```python
from build123d import *

# Parameters (mm, degrees)
F1_DEPTH  = 9.398
F1_FACE_W = 97.914338
F1_FACE_H = 9.398
F2_DEPTH  = 25.4


with BuildPart() as f1:
    # F0 (on Top) → F1 (new body)
    with BuildSketch(Plane.XY):
        Polygon((40.420551, 41.290432), (-57.493787, 42.872965), (-57.493787, -29.132366), (40.420551, -29.132366), (40.420551, 27.838886), align=None)
        Polygon((-53.017702, -20.82406), (-53.017702, 36.542833), (34.834471, 34.169026), (34.834471, -22.243964), align=None, mode=Mode.SUBTRACT)
    extrude(amount=-F1_DEPTH)

    # F1_face (on face) → F2 (join)
    with BuildSketch(Plane(origin=(-8.536618, -29.132366, -4.699), x_dir=(1, 0, 0), z_dir=(0, -1, 0))):
        Rectangle(F1_FACE_W, F1_FACE_H)
    extrude(amount=F2_DEPTH)


solid = f1.part
```
Design review of the part built by this model. Coordinates are the model's own, in mm. A direction names the side the tool comes from. Round coordinates to 2 decimals unless told otherwise and drop trailing zeros. Write each loop counter-clockwise with the first axis right and the second up, starting at its lowest first coordinate (ties: lowest second). Pieces come first, ordered by that corner, then holes. Notation, with made-up numbers: (86, 64.25) -> (106, 64.25) arc R27 ccw to (106, 81.25) -> close; hole circle Ø11 at (-5.75, 29.5). An arc over 180 degrees is marked (long way). Write item = value, one per line. Start each with the question number.
1) Mouldability with a two-part tool opening along Y and no side actions: class faces 3 (the face through (-57.494, -5, -5)), 4 (the face through (-9, -54.532, -5)), 5 (the face through (-53.018, 7, -5)) as +Y half, -Y half, draft (parallel to the pull), parting line (faces both ways), or undercut.
2) Take a section at A-A, the plane z = -2. State the section outline as (x, y) points.
3) Clearance check with flat-ended pins moving along their axes: pin 1 (2 mm diameter, centred on x = 28, z = -3.5, fed in from +Y); pin 2 (5 mm diameter, centred on x = -44, y = -18, fed in from -Z). State where each tip first meets the part, or that it passes through.
4) Tool access review of faces 1 (the face through (34.834, 6, -5)), 2 (the face through (40.421, -6, -5)): name each direction out of +Z, -Z, +X, -X, +Y, -Y from which nothing blocks a thin tool from reaching the whole face with its end or side.
5) Wall thickness on probe 1 along X at (y, z) = (12.5, -8.5); probe 2 along Y at (x, z) = (32.5, -1.5); probe 3 along Y at (x, z) = (29, -3): over which ranges is each line inside the solid? List them lowest first. Write a range as from..to.
6) Take a section at C-C, the plane x = 10. State the section outline as (y, z) points, plus the area to 3 significant figures.
7) Take a section at B-B, the plane y = 10. State the section outline as (x, z) points, plus the area to 3 significant figures.
Results list:
q1.face_3 = draft
q1.face_4 = -Y half
q1.face_5 = undercut
q2.outline = (-57.49, -54.53) -> (40.42, -54.53) -> (40.42, 41.29) -> (-57.49, 42.87) -> close; hole (-53.02, -20.82) -> (34.83, -22.24) -> (34.83, 34.17) -> (-53.02, 36.54) -> close
q3.pin_1 = 41.51
q3.pin_2 = through
q4.face_1 = +Z, -Z
q4.face_2 = +Z, -Z, +X, +Y, -Y
q5.probe_1 = -57.49..-53.02, 34.83..40.42
q5.probe_2 = -54.53..-22.21, 34.23..41.42
q5.probe_3 = -54.53..-22.15, 34.33..41.48
q6.outline = (-54.53, -9.4) -> (-21.84, -9.4) -> (-21.84, 0) -> (-54.53, 0) -> close; (34.84, -9.4) -> (41.78, -9.4) -> (41.78, 0) -> (34.84, 0) -> close
q6.area = 372 mm²
q7.outline = (-57.49, -9.4) -> (-53.02, -9.4) -> (-53.02, 0) -> (-57.49, 0) -> close; (34.83, -9.4) -> (40.42, -9.4) -> (40.42, 0) -> (34.83, 0) -> close
q7.area = 94.6 mm²
